Geometry: final body of the model. Coordinates: model frame, mm. Give positions to 0.01 mm unless a question says otherwise; leave off trailing zeros. Write each loop counter-clockwise with the first axis right and the second up, starting at its lowest first coordinate (ties: lowest second). Pieces come first, ordered by that corner, then holes. Notation, with made-up numbers: (67, -15) -> (103, -15) arc R12 ccw to (103, 4) -> close; hole circle Ø11 at (36.25, 69). An arc over 180 degrees is marked (long way). Answer as a JSON object with one key per item and string values. Group by question number.
(1) Section query A-A on y = -403.5. Output: boundary loops of the cut face in (x, z), plus the area to 3 significant figures.
(2) Contact query for flat-ended pins moving along their axis: pin 1 Ø10 at (y, z) = (-405.5, -564.5) entering from -X; pin 2 Ø4 at (x, y) = (-8.5, -388.5) entering from +Z; pin 3 Ø1.5 at (x, z) = (33, -603) entering from +Y. Output: stop coordinate, or through.
(3) Material intervals for probe 1 along Y at (x, z) = (85.5, -560); probe 2 along Y at (x, z) = (-10, -587); probe 3 along Z at (x, y) = (7.5, -398), sorted ascending.
(4) Section query B-B on x = 62. Output: boundary loops of the cut face in (y, z).
from build123d import *

# Parameters (mm, degrees)
BOSS_EXTRUDE1_DEPTH = 0.0762


with BuildPart() as part:
    # Sketch2 → Boss-Extrude1 (new, symmetric)
    with BuildSketch(Plane(origin=(-109.649906409, -282.836957695, -713.595872526), x_dir=(0.998460453708484, 0.05529862010587768, 0.004334165967541292), z_dir=(0.04480550370073853, -0.7579973701260059, -0.6507168767752854))):
        with BuildLine():
            Line((40.522667634, 135.902493489), (198.13852487, 135.902493489))
            add(Edge.make_bspline(
                [(235, 127.150580223), (217.608315086, 135.902493489), (198.13852487, 135.902493489)],
                knots=[1.10455701, 1.10455701, 1.10455701, 1.570796327, 1.570796327, 1.570796327], degree=2, weights=[1, 0.972950446, 1]))
            Line((235, 127.150580223), (235, 287.108094093))
            Line((235, 287.108094093), (40.522667634, 135.902493489))
        make_face()
    extrude(amount=BOSS_EXTRUDE1_DEPTH, both=True)


solid = part.part
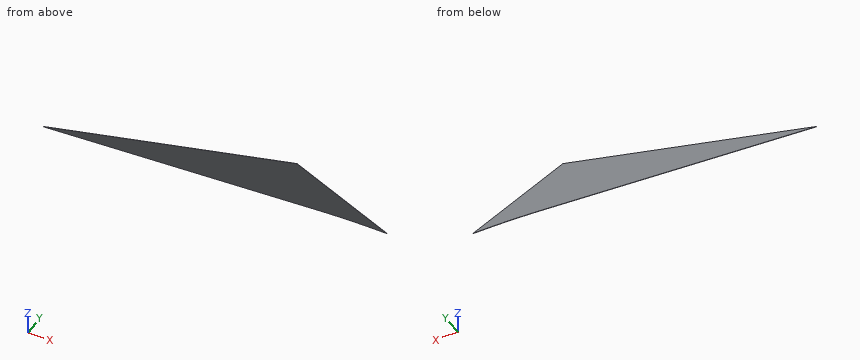
Answer list:
{
 "1": {"outline": "(13.8, -564.66) -> (131.71, -556.54) -> (131.71, -556.3) -> (14.06, -564.4) -> close", "area": "27.6 mm2"},
 "2": {"pin 1": "x = 9.08", "pin 2": "z = -581.1", "pin 3": "y = -368.6"},
 "3": {"probe 1": "-403.26 to -403.06", "probe 2": "-385.73 to -385.52", "probe 3": "-571.5 to -571.26"},
 "4": {"outline": "(-424.68, -536.66) -> (-361.96, -609.73) -> (-361.84, -609.63) -> (-424.57, -536.56) -> close"}
}
